The listing builds one solid part. Answer for the finished solid, in the listing's coordinates (mm). Round coordinates to 2 decimals unless told otherwise and drop trailing zeros. Write each loop counter-clockwise with the first axis right and the second up, starting at its lowest first coordinate (ties: lowest second). Pieces come first, ordered by that corner, then holes. Notation, with made-up numbers: (2.5, 80.5) - (15.5, 80.5) arc R25 ccw to (15.5, 101.5) - close; hole circle Ø8 at (14.5, -2). An arc over 180 degrees is marked (long way). Answer in a Markdown table with one row per item.
from build123d import *

# Parameters (mm, degrees)
SKETCH1_R                   = 1.25
BOSS_EXTRUDE1_DEPTH         = 16.7
F_1_4_28_TAPPED_HOLE1_D     = 3
F_1_4_28_TAPPED_HOLE1_DEPTH = 16


with BuildPart() as part:
    # Sketch1 → Boss-Extrude1 (new body, symmetric)
    with BuildSketch(Plane.XY):
        Polygon((-7.216878365, -6.5), (7.216878365, -6.5), (10.969655115, 0), (5.484827557, 9.5), (-5.484827557, 9.5), (-10.969655115, 0), align=None)
        with Locations((-5, 0)):
            Circle(SKETCH1_R, mode=Mode.SUBTRACT)
        with Locations((5, 0)):
            Circle(SKETCH1_R, mode=Mode.SUBTRACT)
    extrude(amount=BOSS_EXTRUDE1_DEPTH, both=True)

    # 1/4-28 Tapped Hole1
    with Locations(Plane(origin=(0, 9.5, 0), x_dir=(1, 0, 0), z_dir=(0, 1, 0))):
        with Locations((0, 0)):
            Hole(F_1_4_28_TAPPED_HOLE1_D / 2, depth=F_1_4_28_TAPPED_HOLE1_DEPTH)


solid = part.part
(1) Section B-B (x = 4.25) is taken. Give the vertices of the cut face in (y, z), and give its area (3 significant figures).
Checked values:
| item | result |
|---|---|
| outline | (-6.5, -16.7) - (-1, -16.7) - (-1, 16.7) - (-6.5, 16.7) - close; (1, -16.7) - (9.5, -16.7) - (9.5, 16.7) - (1, 16.7) - close |
| area | 468 mm2 |
(2) Section A-A (z = 0) is taken. Give the vertices of the cut face in (x, y), and give its area (3 significant figures).
Checked values:
| item | result |
|---|---|
| outline | (-10.97, 0) - (-7.22, -6.5) - (-1.5, -6.5) - (-1.5, 9.5) - (-5.48, 9.5) - close; (1.5, -6.5) - (7.22, -6.5) - (10.97, 0) - (5.48, 9.5) - (1.5, 9.5) - close; hole circle Ø2.5 at (-5, 0); hole circle Ø2.5 at (5, 0) |
| area | 217 mm2 |
(3) Section C-C (z = -6) is taken. Give the vertices of the cut face in (x, y).
Checked values:
| item | result |
|---|---|
| outline | (-10.97, 0) - (-7.22, -6.5) - (7.22, -6.5) - (10.97, 0) - (5.48, 9.5) - (-5.48, 9.5) - close; hole circle Ø2.5 at (-5, 0); hole circle Ø2.5 at (5, 0) |
(4) Find the intervals of material crossed by line 1 (Y direction, x = 5, z = -3); line 2 (Z direction, x = 0, y = 1.75); line 3 (X direction, y = -0.5, z = 7.5), in increasing order.
Checked values:
| item | result |
|---|---|
| line 1 | y = -6.5 to -1.25, 1.25 to 9.5 |
| line 2 | z = -16.7 to -1.5, 1.5 to 16.7 |
| line 3 | x = -10.68 to -6.15, -3.85 to 3.85, 6.15 to 10.68 |
(5) Section D-D (y = 6) is taken. Give the vertices of the cut face in (x, z).
Checked values:
| item | result |
|---|---|
| outline | (-7.51, -16.7) - (7.51, -16.7) - (7.51, 16.7) - (-7.51, 16.7) - close; hole circle Ø3 at (0, 0) |
(6) For a pull along X with two mould halves and no side action, classify faces 1 (the flat face through (0, 2, -16.7)), 2 (the cylindrical face through (3.75, 0.05, -0.23)), 3 (the flat face through (-8.2, 4.8, 0.2)), 4 (the flat face through (8.266, 4.684, 0.234)) as pulls with the +X half, pulls with the -X half, needs draft (parallel to the pull), parting line crosses it, or undercut.
Checked values:
| item | result |
|---|---|
| face 1 | needs draft |
| face 2 | undercut |
| face 3 | pulls with the -X half |
| face 4 | pulls with the +X half |
(7) Flat-ended cylindrical pins translate along their axes: pin 1 (1.5 mm diameter, centred on y = -4, z = 4, fed in from +X); pin 2 (1 mm diameter, centred on y = 7, z = -0.5, fed in from -X). Find the tip coordinate at first contact, or state that the pin passes through.
Checked values:
| item | result |
|---|---|
| pin 1 | stops at x = 9.09 |
| pin 2 | stops at x = -7.22 |
